from build123d import *

# Parameters (mm, degrees)
SKETCH_1_W          = 36
SKETCH_1_H          = 42
EXTRUDE_1_DEPTH     = 2
EXTRUDE_2_DEPTH     = 9.5
EXTRUDE_3_DEPTH     = 10.5
CUT_EXTRUDE_1_REACH = 3.5
SKETCH_4_R          = 1.75
SKETCH_4_R_2        = 1.3
EXTRUDE_4_DEPTH     = 3.9
CUT_EXTRUDE_2_REACH = 4
SKETCH_4_2_R        = 1.3
SKETCH_5_R          = 2.5
CUT_EXTRUDE_3_DEPTH = 1
SKETCH_6_R          = 2
CUT_EXTRUDE_4_DEPTH = 1.5


with BuildPart() as part:
    # Sketch 1 → Extrude 1 (new body)
    with BuildSketch(Plane.XY):
        with Locations((3, 0)):
            Rectangle(SKETCH_1_W, SKETCH_1_H)
    extrude(amount=EXTRUDE_1_DEPTH)

    # Sketch 2 → Extrude 2 (add)
    with BuildSketch(Plane(origin=(0, 0, 0), x_dir=(-1, 0, 0), z_dir=(0, 0, -1))):
        Polygon((15, -21), (15, 21), (11, 21), (11, 19.75), (14, 19.75), (14, -19.75), (11, -19.75), (11, -21), align=None)
        Polygon((14, 19.75), (11, 19.75), (11, 18.5), (13.5, 18.5), (13.5, -18.5), (11, -18.5), (11, -19.75), (14, -19.75), align=None)
    extrude(amount=EXTRUDE_2_DEPTH)

    # Sketch 2_3 → Extrude 3 (add)
    with BuildSketch(Plane(origin=(0, 0, 0), x_dir=(-1, 0, 0), z_dir=(0, 0, -1))):
        Polygon((14, 19.75), (11, 19.75), (11, 18.5), (13.5, 18.5), (13.5, -18.5), (11, -18.5), (11, -19.75), (14, -19.75), align=None)
    extrude(amount=EXTRUDE_3_DEPTH)

    # Sketch 3 → Cut-Extrude 1 (cut, up to next)
    with BuildSketch(Plane(origin=(-13.5, 0, 0), x_dir=(0, 0, -1), z_dir=(1, 0, 0)), mode=Mode.PRIVATE) as cut_extrude_1_sk1:
        with BuildLine():
            Line((2.35, -3.4), (2.35, 3.4))
            ThreePointArc((2.35, 3.4), (3.95, 5), (5.55, 3.4))
            Line((5.55, 3.4), (5.55, -3.4))
            ThreePointArc((5.55, -3.4), (3.95, -5), (2.35, -3.4))
        make_face()
    cut_extrude_1_tool1 = extrude(cut_extrude_1_sk1.sketch, amount=-CUT_EXTRUDE_1_REACH, mode=Mode.PRIVATE) & part.part
    add(cut_extrude_1_tool1.solids().sort_by_distance((-13.5, 0, -3.95))[0], mode=Mode.SUBTRACT)

    # Sketch 4 → Extrude 4 (add)
    with BuildSketch(Plane(origin=(0, 0, 0), x_dir=(-1, 0, 0), z_dir=(0, 0, -1))):
        with Locations((11, -15.5)):
            Circle(SKETCH_4_R)
        with Locations((11, -15.5)):
            Circle(SKETCH_4_R_2, mode=Mode.SUBTRACT)
        with Locations((-11, 15.5)):
            Circle(SKETCH_4_R)
        with Locations((-11, 15.5)):
            Circle(SKETCH_4_R_2, mode=Mode.SUBTRACT)
    extrude(amount=EXTRUDE_4_DEPTH)

    # Sketch 4_2 → Cut-Extrude 2 (cut, up to next)
    with BuildSketch(Plane(origin=(0, 0, 0), x_dir=(-1, 0, 0), z_dir=(0, 0, -1)), mode=Mode.PRIVATE) as cut_extrude_2_sk1:
        with Locations((11, -15.5)):
            Circle(SKETCH_4_2_R)
    cut_extrude_2_tool1 = extrude(cut_extrude_2_sk1.sketch, amount=-CUT_EXTRUDE_2_REACH, mode=Mode.PRIVATE) & part.part
    add(cut_extrude_2_tool1.solids().sort_by_distance((-11, -15.5, 0))[0], mode=Mode.SUBTRACT)
    # Sketch 4_2 → Cut-Extrude 2 (cut, up to next)
    with BuildSketch(Plane(origin=(0, 0, 0), x_dir=(-1, 0, 0), z_dir=(0, 0, -1)), mode=Mode.PRIVATE) as cut_extrude_2_sk2:
        with Locations((-11, 15.5)):
            Circle(SKETCH_4_2_R)
    cut_extrude_2_tool2 = extrude(cut_extrude_2_sk2.sketch, amount=-CUT_EXTRUDE_2_REACH, mode=Mode.PRIVATE) & part.part
    add(cut_extrude_2_tool2.solids().sort_by_distance((11, 15.5, 0))[0], mode=Mode.SUBTRACT)

    # Sketch 5 → Cut-Extrude 3 (cut)
    with BuildSketch(Plane.XY.offset(2)):
        with Locations((11, 15.5)):
            Circle(SKETCH_5_R)
        with Locations((-11, -15.5)):
            Circle(SKETCH_5_R)
    extrude(amount=-CUT_EXTRUDE_3_DEPTH, mode=Mode.SUBTRACT)

    # Sketch 6 → Cut-Extrude 4 (cut)
    with BuildSketch(Plane(origin=(0, 0, 0), x_dir=(-1, 0, 0), z_dir=(0, 0, -1))):
        with Locations((-8.15, 0)):
            Circle(SKETCH_6_R)
    extrude(amount=-CUT_EXTRUDE_4_DEPTH, mode=Mode.SUBTRACT)


solid = part.part
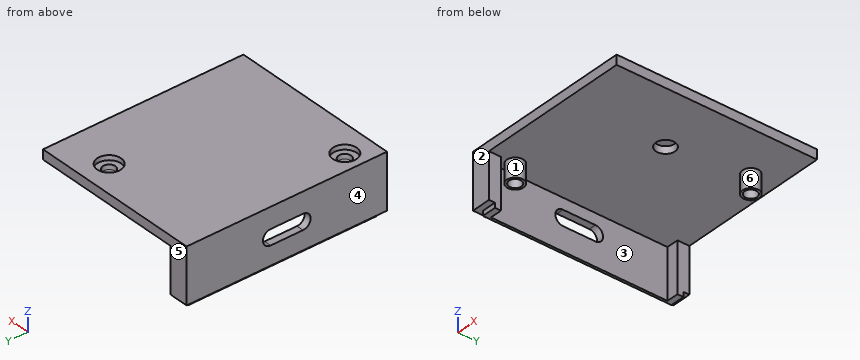
Geometry check sheet. Reference: the model listing, model coordinates, mm. Face numbers are marked on the shaded views. A direction names the side the tool comes from. Round coordinates to 2 decimals unless told otherwise and drop trailing zeros. Write each loop counter-clockwise with the first axis right and the second up, starting at its lowest first coordinate (ties: lowest second). Pieces come first, ordered by that corner, then holes. Notation, with made-up numbers: (-2, -22.75) - (4, -22.75) arc R4 ccw to (4, -16.75) - close; hole circle Ø10 at (58, 41.5). An arc over 180 degrees is marked (long way). One line per item, written item: value.
1. Cross-section at C-C on y = 15.5. Record the boundary of the cut face in (x, z).
The answers:
outline: (-15, -9.5) - (-14, -9.5) - (-14, -10.5) - (-13.5, -10.5) - (-13.5, 0) - (9.25, 0) - (9.25, -3.9) - (9.7, -3.9) - (9.7, 1) - (8.5, 1) - (8.5, 2) - (-15, 2) - close; (12.3, -3.9) - (12.75, -3.9) - (12.75, 0) - (21, 0) - (21, 2) - (13.5, 2) - (13.5, 1) - (12.3, 1) - close
2. Set-up check for the marked faces 1 and 2: record each of +Z, -Z, +X, -X, +Y, -Y from which the full face is reachable in a straight line by a thin tool's end or side.
The answers:
face 1: -Z
face 2: +Z, -Z, +X, -X, -Y
3. Depth check by flat-ended pin: pin 1 Ø6.5 at (x, y) = (8.15, 0) entering from -Z; pin 2 Ø4 at (x, y) = (-11, -15.5) entering from +Z; pin 3 Ø8 at (x, y) = (9.5, 15) entering from -Z; pin 4 Ø8 at (x, y) = (-11, -15.5) entering from -Z. Enter the tip coordinate at first touch or a pass-through.
The answers:
pin 1: stops at z = 0
pin 2: stops at z = 1
pin 3: stops at z = -3.9
pin 4: stops at z = -10.5
4. Scan lines: L1, parallel to Y at x = 11, z = 0.3; L2, parallel to Y at x = 11, z = -2.6; L3, parallel to Z at x = -2, y = -8. Record each from-to range of solid material in increasing order.
The answers:
L1: y = -21 to 14.2, 16.8 to 21
L2: y = 13.75 to 14.2, 16.8 to 17.25
L3: z = 0 to 2
5. Cross-section at A-A on z = -0.5. Record the boundary of the cut face in (x, y), and give its area (3 significant figures).
The answers:
outline: (-15, -21) - (-11, -21) - (-11, -18.5) - (-13.5, -18.5) - (-13.5, 18.5) - (-11, 18.5) - (-11, 21) - (-15, 21) - close; circle Ø3.5 at (-11, -15.5); circle Ø3.5 at (11, 15.5); hole circle Ø2.6 at (-11, -15.5); hole circle Ø2.6 at (11, 15.5)
area: 84.1 mm^2
6. Cross-section at B-B on x = 11. Record the boundary of the cut face in (y, z).
The answers:
outline: (-21, 0) - (13.75, 0) - (13.75, -3.9) - (14.2, -3.9) - (14.2, 1) - (13, 1) - (13, 2) - (-21, 2) - close; (16.8, -3.9) - (17.25, -3.9) - (17.25, 0) - (21, 0) - (21, 2) - (18, 2) - (18, 1) - (16.8, 1) - close
7. Cross-section at D-D on y = 9.5. Record the boundary of the cut face in (x, z).
The answers:
outline: (-15, -9.5) - (-14, -9.5) - (-14, -10.5) - (-13.5, -10.5) - (-13.5, 0) - (21, 0) - (21, 2) - (-15, 2) - close
8. Mould release check, pull along Y, two halves, no side actions. Record for the marked faces 3, 4, 5 and 6: released by +Y, released by -Y, zero draft, split by the parting line, or undercut.
The answers:
face 3: undercut
face 4: zero draft
face 5: released by +Y
face 6: split by the parting line
